from build123d import *

# Parameters (mm, degrees)
SKETCH_2_W          = 116.6
SKETCH_2_H          = 20.43
EXTRUDE_1_DEPTH     = 25.5
CUT_EXTRUDE_1_DEPTH = 5
M5X0_81_D           = 4.2
HOLE_WIZARD_6_0_1_D = 6
CHAMFER_1_SIZE      = 0.5


with BuildPart() as part:
    # Эскиз2 → Бобышка-Вытянуть1 (new body)
    with BuildSketch(Plane.XY):
        with Locations((58.3, 10.215)):
            Rectangle(SKETCH_2_W, SKETCH_2_H)
    extrude(amount=-EXTRUDE_1_DEPTH)

    # Эскиз1 → Вырез-Вытянуть1 (cut)
    with BuildSketch(Plane.XY):
        Polygon((27.35, 17.73), (29.05, 19.43), (30.75, 17.73), (44.75, 17.73), (46.45, 19.43), (48.15, 17.73), (62.15, 17.73), (63.85, 19.43), (65.55, 17.73), (79.55, 17.73), (81.25, 19.43), (82.95, 17.73), (96.95, 17.73), (98.65, 19.43), (100.35, 17.73), (110.3, 17.73), (110.3, 0), (0, 0), (0, 17.73), (9.95, 17.73), (11.65, 19.43), (13.35, 17.73), align=None)
    extrude(amount=-CUT_EXTRUDE_1_DEPTH, mode=Mode.SUBTRACT)

    # Отверстие обработанное метчиком M5x0.81 (through all)
    with Locations(Plane(origin=(-38.872854219, 5.478694599, -5), x_dir=(1, 0, 0), z_dir=(0, 0, 1))):
        with Locations((94.022854219, 4.751305401), (49.022854219, 4.751305401), (139.022854219, 4.751305401)):
            Hole(M5X0_81_D / 2)

    # Отверстия под штифты Ø6.0 мм1 (through all)
    with Locations(Plane.XY.offset(-5)):
        with Locations((32.65, 10.23), (77.65, 10.23)):
            Hole(HOLE_WIZARD_6_0_1_D / 2)

    # Фаска1
    chamfer_1_edges = [part.edges().sort_by_distance(p)[0] for p in [
        (116.6, 10.215, -25.5),
        (58.3, 20.43, -25.5),
        (0, 10.215, -25.5),
        (58.3, 0, -25.5),
        (0, 20.43, -12.75),
        (116.6, 20.43, -12.75),
        (116.6, 0, -12.75),
        (0, 0, -15.25),
    ]]
    chamfer(chamfer_1_edges, length=CHAMFER_1_SIZE)


solid = part.part
Read the model definition and answer for the solid it produces. Units are mm, in the model's axes. A direction names the side the tool comes from. Coordinates: 2 decimals unless noted, no trailing zeros. Write each loop counter-clockwise with the first axis right and the second up, starting at its lowest first coordinate (ties: lowest second). Pieces come first, ordered by that corner, then holes. Notation, with made-up numbers: (-36, 3) -> (-7, 3) arc R17 ccw to (-7, 33) -> close; hole circle Ø10 at (62, 52.5). An arc over 180 degrees is marked (long way). Return JSON: item names as keys, results as strings.
(1) The part is cut by section A-A on x = 55.15. Give the vertices of the cut face in (y, z), then the cut area to 3 significant figures.
Answers below:
{"outline": "(0, -25) -> (0.5, -25.5) -> (8.13, -25.5) -> (8.13, -5) -> (0, -5) -> close; (12.33, -25.5) -> (19.93, -25.5) -> (20.43, -25) -> (20.43, 0) -> (17.73, 0) -> (17.73, -5) -> (12.33, -5) -> close", "area": "346 mm^2"}
(2) Which of the six approach directions +Z, -Z, +X, -X, +Y, -Y give full straight-line access (tool end or side, diameter ignored) to faces 1 (the flat face through (5, 17.73, -2)), 2 (the cylindrical face through (99.02, 12, -15.39))?
Answers below:
{"face 1": "+Z, -X, -Y", "face 2": "+Z, -Z"}
(3) The part is cut by section B-B on y = 10.23. Give the vertices of the cut face in (x, z).
Answers below:
{"outline": "(0, -25) -> (0.5, -25.5) -> (8.05, -25.5) -> (8.05, -5) -> (0, -5) -> close; (12.25, -25.5) -> (29.65, -25.5) -> (29.65, -5) -> (12.25, -5) -> close; (35.65, -25.5) -> (53.05, -25.5) -> (53.05, -5) -> (35.65, -5) -> close; (57.25, -25.5) -> (74.65, -25.5) -> (74.65, -5) -> (57.25, -5) -> close; (80.65, -25.5) -> (98.05, -25.5) -> (98.05, -5) -> (80.65, -5) -> close; (102.25, -25.5) -> (116.1, -25.5) -> (116.6, -25) -> (116.6, 0) -> (110.3, 0) -> (110.3, -5) -> (102.25, -5) -> close"}
(4) For a pull along X with two mould halves and no side action, classify faces 3 (the cylindrical face through (29.79, 11.13, -15.39)), 4 (the flat face through (105, 17.73, -2)), 5 (the flat face through (116.6, 10, -12)), 6 (the cylindrical face through (74.79, 11.13, -15.39)) as pulls with the +X half, pulls with the -X half, needs draft (parallel to the pull), parting line crosses it, or undercut.
Answers below:
{"face 3": "undercut", "face 4": "needs draft", "face 5": "pulls with the +X half", "face 6": "undercut"}
(5) The part is cut by section C-C on z = -9. Give the vertices of the cut face in (x, y).
Answers below:
{"outline": "(0, 0.5) -> (0.5, 0) -> (116.1, 0) -> (116.6, 0.5) -> (116.6, 19.93) -> (116.1, 20.43) -> (0.5, 20.43) -> (0, 19.93) -> close; hole circle Ø4.2 at (10.15, 10.23); hole circle Ø6 at (32.65, 10.23); hole circle Ø4.2 at (55.15, 10.23); hole circle Ø6 at (77.65, 10.23); hole circle Ø4.2 at (100.15, 10.23)"}
(6) The part is cut by section D-D on y = 15. Give the vertices of the cut face in (x, z), then the cut area to 3 significant figures.
Answers below:
{"outline": "(0, -25) -> (0.5, -25.5) -> (116.1, -25.5) -> (116.6, -25) -> (116.6, 0) -> (110.3, 0) -> (110.3, -5) -> (0, -5) -> close", "area": "2,420 mm^2"}
(7) Consider line 1 along X through (y, z) = (13, -9); line 2 along Y through (x, z) = (32.65, -10.75); line 3 along Y through (x, z) = (55.15, -17.5). Determine where each line is inside the solid, lowest interval first. Write a range as from..to.
Answers below:
{"line 1": "0..31.5, 33.8..76.5, 78.8..116.6", "line 2": "0..7.23, 13.23..20.43", "line 3": "0..8.13, 12.33..20.43"}
(8) Each of these flat-tipped pins is pushed along its axis until it touches: P1, Ø3.5, axis at x = 32.65, y = 10.23, coming from the +Z side; P2, Ø1, axis at x = 93, y = 16, coming from the +Z side; P3, Ø4, axis at x = 74, z = -2, coming from the -Y side; P4, Ø1.5, axis at y = 5.5, z = -1.5, coming from the -X side. Where does it stop, or does it pass through?
Answers below:
{"P1": "through", "P2": "z = -5", "P3": "y = 17.73", "P4": "x = 110.3"}
